```python
from build123d import *

# Parameters (mm, degrees)
EXTUDEMAIN_DEPTH = 2.75
PIHOLES_REACH    = 29.328
SKETCH2_R        = 1.1


with BuildPart() as part:
    # Main → ExtudeMain (new body)
    with BuildSketch(Plane(origin=(0, 0, 0), x_dir=(1, 0, 0), z_dir=(0, 1, 0))):
        with BuildLine():
            Line((-19.267949192, 1), (-1.732050808, 1))
            ThreePointArc((-1.732050808, 1), (-1.414213562, 1.414213562), (-1, 1.732050808))
            Line((-1, 1.732050808), (-1, 10.767949192))
            ThreePointArc((-1, 10.767949192), (0, 14.5), (1, 10.767949192))
            Line((1, 10.767949192), (1, 1.732050808))
            ThreePointArc((1, 1.732050808), (1.414213562, -1.414213562), (-1.732050808, -1))
            Line((-1.732050808, -1), (-19.267949192, -1))
            ThreePointArc((-19.267949192, -1), (-22.414213562, -1.414213562), (-22, 1.732050808))
            Line((-22, 1.732050808), (-22, 10.767949192))
            ThreePointArc((-22, 10.767949192), (-21, 14.5), (-20, 10.767949192))
            Line((-20, 10.767949192), (-20, 1.732050808))
            ThreePointArc((-20, 1.732050808), (-19.585786438, 1.414213562), (-19.267949192, 1))
        make_face()
    extrude(amount=EXTUDEMAIN_DEPTH)

    # Sketch2 → PiHoles (cut, up to next)
    with BuildSketch(Plane(origin=(0, 2.75, 0), x_dir=(1, 0, 0), z_dir=(0, 1, 0)), mode=Mode.PRIVATE) as piholes_sk1:
        with Locations(Location((-21, 12.5, 0), (0, 0, 270))):
            Circle(SKETCH2_R)
    piholes_tool1 = extrude(piholes_sk1.sketch, amount=-PIHOLES_REACH, mode=Mode.PRIVATE) & part.part
    # Sketch2 → PiHoles (cut, up to next)
    with BuildSketch(Plane(origin=(0, 2.75, 0), x_dir=(1, 0, 0), z_dir=(0, 1, 0)), mode=Mode.PRIVATE) as piholes_sk2:
        with Locations(Location((0, 12.5, 0), (0, 0, 270))):
            Circle(SKETCH2_R)
    piholes_tool2 = extrude(piholes_sk2.sketch, amount=-PIHOLES_REACH, mode=Mode.PRIVATE) & part.part
    # Sketch2 → PiHoles (cut, up to next)
    with BuildSketch(Plane(origin=(0, 2.75, 0), x_dir=(1, 0, 0), z_dir=(0, 1, 0)), mode=Mode.PRIVATE) as piholes_sk3:
        with Locations(Location((0, 0, 0), (0, 0, 270))):
            Circle(SKETCH2_R)
    piholes_tool3 = extrude(piholes_sk3.sketch, amount=-PIHOLES_REACH, mode=Mode.PRIVATE) & part.part
    # Sketch2 → PiHoles (cut, up to next)
    with BuildSketch(Plane(origin=(0, 2.75, 0), x_dir=(1, 0, 0), z_dir=(0, 1, 0)), mode=Mode.PRIVATE) as piholes_sk4:
        with Locations(Location((-21, 0, 0), (0, 0, 270))):
            Circle(SKETCH2_R)
    piholes_tool4 = extrude(piholes_sk4.sketch, amount=-PIHOLES_REACH, mode=Mode.PRIVATE) & part.part
    add(piholes_tool1.solids().sort_by_distance((-21, 2.75, -12.5))[0], mode=Mode.SUBTRACT)
    add(piholes_tool2.solids().sort_by_distance((0, 2.75, -12.5))[0], mode=Mode.SUBTRACT)
    add(piholes_tool3.solids().sort_by_distance((0, 2.75, 0))[0], mode=Mode.SUBTRACT)
    add(piholes_tool4.solids().sort_by_distance((-21, 2.75, 0))[0], mode=Mode.SUBTRACT)


solid = part.part
```
Geometry: final body of the model. Coordinates: model frame, mm. A direction names the side the tool comes from. Coordinates: 2 decimals unless noted, no trailing zeros. Order: outer loops, then holes, each group sorted by start corner. A loop starts at its lowest first (then second) coordinate and runs counter-clockwise, first axis right, second up. Notation, with made-up numbers: (-2, 72.5) - (50, 72.5) arc R17 ccw to (50, 103.5) - close; hole circle Ø1 at (23, 41). An arc over 180 degrees is marked (long way). Write each question's results on one line, items separated by ' | '.
1) Set-up query: faces 1 (the flat face through (1, 1, -6)), 2 (the flat face through (-10, 1, 1)), 3 (the flat face through (-20, 1, -6)). Return all of +Z, -Z, +X, -X, +Y, -Y with unobstructed straight access to the full face (end or side cutting, diameter ignored); none if empty.
Results list:
face 1: +X, +Y, -Y | face 2: +Z, +Y, -Y | face 3: +Y, -Y
2) Section C-C, the plane y = 2.3. Return loops of the section in (x, z), plus the area to 3 significant figures.
Results list:
outline: (-22, -10.77) arc R2 ccw (long way) to (-20, -10.77) - (-20, -1.73) arc R2 ccw to (-19.27, -1) - (-1.73, -1) arc R2 ccw to (-1, -1.73) - (-1, -10.77) arc R2 ccw (long way) to (1, -10.77) - (1, -1.73) arc R2 ccw (long way) to (-1.73, 1) - (-19.27, 1) arc R2 ccw (long way) to (-22, -1.73) - close; hole circle Ø2.2 at (-21, -12.5); hole circle Ø2.2 at (-21, 0); hole circle Ø2.2 at (0, -12.5); hole circle Ø2.2 at (0, 0) | area: 104 mm^2
3) Line query: line 1 (X direction, y = 0.75, z = 0); line 2 (X direction, y = 2.2, z = -7.5); line 3 (X direction, y = 2.25, z = -0.5). Output: solid intervals per line, ascending. Write a range as from..to.
Results list:
line 1: -23..-22.1, -19.9..-1.1, 1.1..2 | line 2: -22..-20, -1..1 | line 3: -22.94..-21.98, -20.02..-0.98, 0.98..1.94
4) Pin query (flat end, axial travel): pin 1 (3 mm diameter, centred on x = -10, z = -2, fed in from +Y); pin 2 (1.4 mm diameter, centred on y = 1.5, z = -7.5, fed in from -X). Return the tip coordinate at first contact, or that it passes through.
Results list:
pin 1: y = 2.75 | pin 2: x = -22
5) Pull-direction query (X, two-part tool) for faces 4 (the cylindrical face through (-22.074, 1.394, -0.238)), 5 (the flat face through (-22, 1, -6)), 6 (the flat face through (-10.4, 2.75, -0.8)); classes: pulls with the +X half, pulls with the -X half, needs draft (parallel to the pull), parting line crosses it, or undercut.
Results list:
face 4: undercut | face 5: pulls with the -X half | face 6: needs draft
6) Section D-D, the plane z = -6.5. Return loops of the section in (x, y).
Results list:
outline: (-22, 0) - (-20, 0) - (-20, 2.75) - (-22, 2.75) - close; (-1, 0) - (1, 0) - (1, 2.75) - (-1, 2.75) - close
7) Section B-B, the plane x = 0. Return loops of the section in (y, z).
Results list:
outline: (0, -14.5) - (2.75, -14.5) - (2.75, -13.6) - (0, -13.6) - close; (0, -11.4) - (2.75, -11.4) - (2.75, -1.1) - (0, -1.1) - close; (0, 1.1) - (2.75, 1.1) - (2.75, 2) - (0, 2) - close
8) Section A-A, the plane z = -12.5. Return loops of the section in (x, y).
Results list:
outline: (-23, 0) - (-22.1, 0) - (-22.1, 2.75) - (-23, 2.75) - close; (-19.9, 0) - (-19, 0) - (-19, 2.75) - (-19.9, 2.75) - close; (-2, 0) - (-1.1, 0) - (-1.1, 2.75) - (-2, 2.75) - close; (1.1, 0) - (2, 0) - (2, 2.75) - (1.1, 2.75) - close
